Here's how the part is built. I have some questions about the finished solid (model axes, mm). Face numbers are marked on the shaded views. Round coordinates to 2 decimals unless told otherwise and drop trailing zeros. Order: outer loops, then holes, each group sorted by start corner. A loop starts at its lowest first (then second) coordinate and runs counter-clockwise, first axis right, second up. Notation, with made-up numbers: (55.25, 86) -> (91.25, 86) arc R20 cw to (91.25, 97) -> close; hole circle Ø3 at (47, 54). An arc over 180 degrees is marked (long way). One line per item, written item: value.
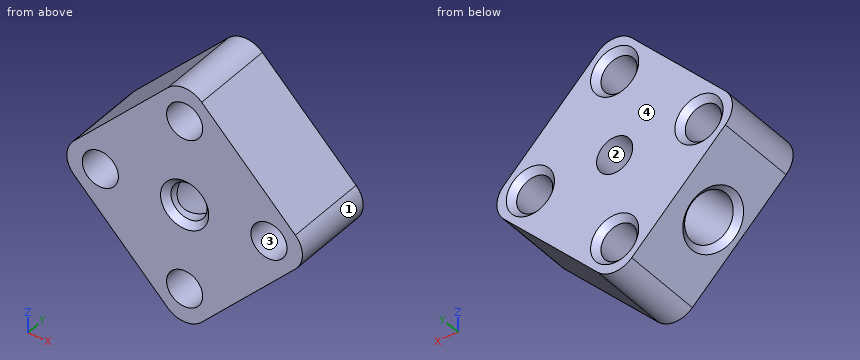
```python
from build123d import *

# Parameters (mm, degrees)
F0_R     = 1.5
F1_DEPTH = 7
F2_R     = 2
F3_DEPTH = 7
F4_SIZE  = 0.5


with BuildPart() as f1:
    # F0 (on Front) → F1 (new body)
    with BuildSketch(Plane.XZ):
        with BuildLine():
            Line((-9.192388, -1.414214), (-1.414214, -9.192388))
            ThreePointArc((-1.414214, -9.192388), (0, -9.778175), (1.414214, -9.192388))
            Line((1.414214, -9.192388), (9.192388, -1.414214))
            ThreePointArc((9.192388, -1.414214), (9.778175, 0), (9.192388, 1.414214))
            Line((9.192388, 1.414214), (1.414214, 9.192388))
            ThreePointArc((1.414214, 9.192388), (0, 9.778175), (-1.414214, 9.192388))
            Line((-1.414214, 9.192388), (-9.192388, 1.414214))
            ThreePointArc((-9.192388, 1.414214), (-9.778175, 0), (-9.192388, -1.414214))
        make_face()
        with Locations((0, -7)):
            Circle(F0_R, mode=Mode.SUBTRACT)
        with Locations((-7, 0)):
            Circle(F0_R, mode=Mode.SUBTRACT)
        Circle(F0_R, mode=Mode.SUBTRACT)
        with Locations((7, 0)):
            Circle(F0_R, mode=Mode.SUBTRACT)
        with Locations((0, 7)):
            Circle(F0_R, mode=Mode.SUBTRACT)
    extrude(amount=F1_DEPTH)

    # F2 (on face) → F3 (cut)
    with BuildSketch(Plane(origin=(-5.303301, 0, -5.303301), x_dir=(0.707107, 0, -0.707107), z_dir=(-0.707107, 0, -0.707107))):
        with Locations((0, 4)):
            Circle(F2_R)
    extrude(amount=-F3_DEPTH, mode=Mode.SUBTRACT)

    # F4
    f4_edges = [f1.edges().sort_by_distance(p)[0] for p in [
        (-1.5, 0, 7),
        (-8.5, 0, 0),
        (-1.5, 0, -7),
        (5.5, 0, 0),
        (-1.5, -7, 0),
        (-6.717514, -4, -3.889087),
    ]]
    chamfer(f4_edges, length=F4_SIZE)


solid = f1.part
```
Q1. I want a section at C-C on z = -1. Give the number of separate pieces and of enclosed holes in the cut face, then the cut area to 3 significant figures.
Answers:
separate pieces: 4
enclosed holes: 0
area: 76.8 mm2
Q2. I want a section at B-B on x = 7. Write out the boundary of the cut face in (y, z).
Answers:
outline: (-7, -3.61) -> (0, -3.61) -> (0, -2) -> (-0.5, -1.5) -> (-7, -1.5) -> close; (-7, 1.5) -> (-0.5, 1.5) -> (0, 2) -> (0, 3.61) -> (-7, 3.61) -> close
Q3. I need wall thicknesses on line 1 along Z through (x, y) = (0, -2); line 2 along Z through (x, y) = (-0.25, -4.5); line 3 along X through (y, z) = (-2.5, -0.25). Which ranges of each line are inside material? Lowest first, please.
Answers:
line 1: -9.78 to -8.5, -5.5 to -1.5, 1.5 to 5.5, 8.5 to 9.78
line 2: -9.76 to -8.48, -5.52 to -2.99, 1.48 to 5.52, 8.48 to 9.76
line 3: -9.76 to -8.48, -5.52 to -2.12, 1.48 to 5.52, 8.48 to 9.76
Q4. I want a section at A-A on y = -1. Write out the boundary of the cut face in (x, z), then the cut area to 3 significant figures.
Answers:
outline: (-9.19, -1.41) -> (-1.41, -9.19) arc R2 ccw to (1.41, -9.19) -> (9.19, -1.41) arc R2 ccw to (9.19, 1.41) -> (1.41, 9.19) arc R2 ccw to (-1.41, 9.19) -> (-9.19, 1.41) arc R2 ccw to start; hole circle Ø3 at (-7, 0); hole circle Ø3 at (0, -7); hole circle Ø3 at (0, 0); hole circle Ø3 at (0, 7); hole circle Ø3 at (7, 0)
area: 186 mm2
Q5. For P1, Ø6, axis at x = 6, z = 1, coming from the -Y side; P2, Ø1.8, axis at x = 0, z = 7, coming from the +Y side (1 decimal); P3, Ø1, axis at x = 2.5, y = -1, coming from the +Z side; P4, Ø1.5, axis at x = -7, y = -4.5, coming from the -Z side, each with a flat end and sliding along its axis, tell me the tip position at first contact or that it passes through.
Answers:
P1: y = -7
P2: through
P3: z = 8.61
P4: z = -3.77
Q6. If we mould it in two halves opening along Z, with no side actions, what happens to the marked faces 1, 2, 3 and 4? For each: pulls with the +Z half, pulls with the -Z half, needs draft (parallel to the pull), parting line crosses it, or undercut.
Answers:
face 1: parting line crosses it
face 2: undercut
face 3: undercut
face 4: needs draft
